Geometry: final body of the model. Coordinates: model frame, mm. Coordinates: 2 decimals unless noted, no trailing zeros. Loops run counter-clockwise (first coordinate to the right, second up) from the corner with the lowest first, then second, coordinate; pieces in that order, holes last. Notation, with made-up numbers: (46.5, -37.5) - (82.5, -37.5) arc R9 cw to (82.5, -31.5) - close; hole circle Ø6 at (-22.5, 54). An arc over 180 degrees is marked (long way). Answer in a Markdown table with one row per item.
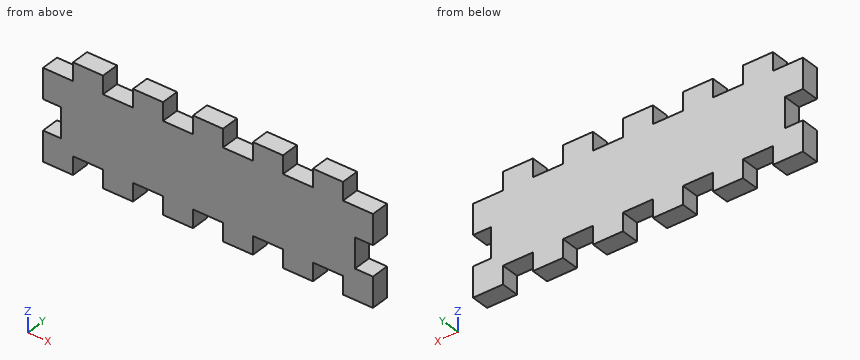
Autodesk Inventor part; units mm, degrees
ref_plane "YZ Plane" through (0, 0, 0) normal (1, 0, 0) x (0, 1, 0)
ref_plane "XZ Plane" through (0, 0, 0) normal (0, 1, 0) x (-1, 0, 0)
ref_plane "XY Plane" through (0, 0, 0) normal (0, 0, 1) x (1, 0, 0)
sketch "Skizze1" plane through (0, 0, 0) normal (0, 1, 0) x (-1, 0, 0)
  line L0 (-5, 0) -> (-5, -3)
  line L1 (-5, -3) -> (0, -3)
  line L2 (-5, 0) -> (-10, 0)
  line L3 (-10, 0) -> (-10, -3)
  line L4 (-10, -3) -> (-15, -3)
  line L5 (-15, 0) -> (-15, -3)
  line L6 (-15, 0) -> (-20, 0)
  line L7 (-20, 0) -> (-20, -3)
  line L8 (-20, -3) -> (-25, -3)
  line L9 (-25, 0) -> (-25, -3)
  line L10 (-25, 0) -> (-30, 0)
  line L11 (-30, 0) -> (-30, -3)
  line L12 (-30, -3) -> (-35, -3)
  line L13 (-35, 0) -> (-35, -3)
  line L14 (-35, 0) -> (-40, 0)
  line L15 (-40, 0) -> (-40, -3)
  line L16 (-40, -3) -> (-45, -3)
  line L17 (-45, 0) -> (-45, -3)
  line L18 (-45, 0) -> (-50, 0)
  line L19 (-50, 0) -> (-50, -3)
  line L20 (-50, -3) -> (-55, -3)
  line L21 (-55, -3) -> (-55, -8)
  line L22 (-55, -8) -> (-52, -8)
  line L23 (-52, -8) -> (-52, -13)
  line L24 (-52, -13) -> (-55, -13)
  line L25 (0, -3) -> (0, -8)
  line L26 (0, -8) -> (-3, -8)
  line L27 (-3, -8) -> (-3, -13)
  line L28 (-3, -13) -> (0, -13)
  line L29 (0, -13) -> (0, -18)
  line L30 (-55, -18) -> (-55, -13)
  line L31 (0, -18) -> (-5, -18)
  line L32 (-5, -18) -> (-5, -15)
  line L33 (-5, -15) -> (-10, -15)
  line L34 (-10, -15) -> (-10, -18)
  line L35 (-20, -15) -> (-20, -18)
  line L36 (-15, -18) -> (-15, -15)
  line L37 (-10, -18) -> (-15, -18)
  line L38 (-15, -15) -> (-20, -15)
  line L39 (-30, -15) -> (-30, -18)
  line L40 (-25, -18) -> (-25, -15)
  line L41 (-20, -18) -> (-25, -18)
  line L42 (-25, -15) -> (-30, -15)
  line L43 (-40, -15) -> (-40, -18)
  line L44 (-35, -18) -> (-35, -15)
  line L45 (-30, -18) -> (-35, -18)
  line L46 (-35, -15) -> (-40, -15)
  line L47 (-50, -15) -> (-50, -18)
  line L48 (-45, -18) -> (-45, -15)
  line L49 (-40, -18) -> (-45, -18)
  line L50 (-45, -15) -> (-50, -15)
  line L51 (-50, -18) -> (-55, -18)
  point P0 (0, 0)
  dimension "d2" = 5
  dimension "d3" = 3
  dimension "d6" = 10
  dimension "d13" = 10
extrude "Extrusion1" add sketch "Skizze1" along normal blind 3
properties part number "plate_front_small" material "Holz (Kirsche)"
(1) Ray query, probe 1 along Z at (x, y) = (17.5, 2); probe 2 along X at (y, z) = (1.6, -10.75); probe 3 along Z at (x, y) = (40.5, 2.05). Return the intervals inside material, ascending.
Verdict:
| item | result |
|---|---|
| probe 1 | z = -15 to 0 |
| probe 2 | x = 3 to 52 |
| probe 3 | z = -18 to -3 |
(2) Cut plane A-A on z = -12. Output: boundary loops of the cut face in (x, y).
Verdict:
| item | result |
|---|---|
| outline | (3, 0) - (52, 0) - (52, 3) - (3, 3) - close |
(3) First-contact query: pin 1 Ø0.9 at (y, z) = (1, -1.5) entering from -X; pin 2 Ø0.9 at (x, y) = (26.5, 2) entering from -Z; pin 3 Ø1.5 at (x, y) = (11.5, 1) entering from +Z. Flat tips, straight axial feed; report the tip coordinate or a pass-through.
Verdict:
| item | result |
|---|---|
| pin 1 | stops at x = 5 |
| pin 2 | stops at z = -15 |
| pin 3 | stops at z = -3 |
(4) Cut plane B-B on x = 13. Output: boundary loops of the cut face in (y, z).
Verdict:
| item | result |
|---|---|
| outline | (0, -18) - (3, -18) - (3, -3) - (0, -3) - close |
